from build123d import *

# Parameters (mm, degrees)
F0_W     = 150
F0_H     = 194.7
F0_R     = 2
F1_DEPTH = 2.032
F2_W     = 20
F2_H     = 2
F3_DEPTH = 35.71875
F4_DEPTH = 66.675
F5_R     = 2
F6_DEPTH = 2
F7_W     = 2.032
F7_H     = 20
F8_DEPTH = 39
F9_R     = 2
F10_R    = 1.99999
F11_R    = 0.5


# Not quite as in the source:
# - a fillet or chamfer is up to 0.001 mm smaller than in the source, because OpenCascade refuses the exact size


with BuildPart() as f1:
    # F0 (on Front) → F1 (new body)
    with BuildSketch(Plane.XZ):
        with Locations((0, -42.35)):
            Rectangle(F0_W, F0_H)
        with Locations((-50, -50)):
            Circle(F0_R, mode=Mode.SUBTRACT)
        with Locations((50, -50)):
            Circle(F0_R, mode=Mode.SUBTRACT)
        with Locations((-37.5, -37.5)):
            Circle(F0_R, mode=Mode.SUBTRACT)
        with Locations((-50, 50)):
            Circle(F0_R, mode=Mode.SUBTRACT)
        with Locations((-37.5, 37.5)):
            Circle(F0_R, mode=Mode.SUBTRACT)
        with Locations((37.5, -37.5)):
            Circle(F0_R, mode=Mode.SUBTRACT)
        with Locations((37.5, 37.5)):
            Circle(F0_R, mode=Mode.SUBTRACT)
        with Locations((50, 50)):
            Circle(F0_R, mode=Mode.SUBTRACT)
    extrude(amount=F1_DEPTH)

    # F2 (on Right) → F3 (join, symmetric)
    with BuildSketch(Plane.YZ):
        with Locations((-12.032, -138.7)):
            Rectangle(F2_W, F2_H)
    extrude(amount=F3_DEPTH, both=True)

    # F2 (on Right) → F4 (join, symmetric)
    with BuildSketch(Plane.YZ):
        Polygon((-24.032, -139.7), (-22.032, -139.7), (-22.032, -137.7), (-22.032, -109.7), (-24.032, -109.7), align=None)
    extrude(amount=F4_DEPTH, both=True)

    # F5 (on face) → F6 (cut, through all)
    with BuildSketch(Plane.XZ.offset(24.032)):
        with Locations((-50.8, -114.7)):
            Circle(F5_R)
        with Locations((-23.6466728747, -130.575)):
            Circle(F5_R)
        with Locations((50.8, -114.7)):
            Circle(F5_R)
        with Locations((23.6466728747, -130.575)):
            Circle(F5_R)
    extrude(amount=-F6_DEPTH, mode=Mode.SUBTRACT)

    # F7 (on face) → F8 (join)
    with BuildSketch(Plane.XY.offset(-137.7)):
        with Locations((-34.70275, -12.032)):
            Rectangle(F7_W, F7_H)
        with Locations((34.70275, -12.032)):
            Rectangle(F7_W, F7_H)
    extrude(amount=F8_DEPTH)

    # F9
    f9_edges = [f1.edges().sort_by_distance(p)[0] for p in [
        (35.71875, -2.032, -119.2),
        (35.71875, -22.032, -124.7),
        (-35.71875, -2.032, -119.2),
        (-35.71875, -22.032, -124.7),
    ]]
    fillet(f9_edges, radius=F9_R)

    # F10 (radius 2 in the source; OpenCascade refuses exactly that, so slightly less here)
    f10_edges = [f1.edges().sort_by_distance(p)[0] for p in [
        (0, 0, -139.7),
        (0, -24.032, -139.7),
    ]]
    fillet(f10_edges, radius=F10_R)

    # F11
    f11_edges = [f1.edges().sort_by_distance(p)[0] for p in [
        (-35.71875, -12.032, -139.7),
        (35.71875, -12.032, -139.7),
        (33.68675, -12.032, -137.7),
        (-33.68675, -12.032, -137.7),
    ]]
    fillet(f11_edges, radius=F11_R)


solid = f1.part
Design review of the part built by this model. Coordinates are the model's own, in mm. A direction names the side the tool comes from. Round coordinates to 2 decimals unless told otherwise and drop trailing zeros. Write each loop counter-clockwise with the first axis right and the second up, starting at its lowest first coordinate (ties: lowest second). Pieces come first, ordered by that corner, then holes. Notation, with made-up numbers: (-28, 77.25) -> (18, 77.25) arc R22 ccw to (18, 108.25) -> close; hole circle Ø9 at (-28, 76). An arc over 180 degrees is marked (long way). One line per item, written item: value. Start each with the question number.
Q1. The part is to be moulded in two halves that separate along Y. For faces 6 (the face through (0, -12, -137.7)), 7 (the face through (1, -24.032, -124)), 8 (the face through (35, -12, -98.7)), say which applies: pulls with the +Y half, pulls with the -Y half, needs draft (parallel to the pull), parting line crosses it, or undercut.
Q2. Add section B-B (z = 37.5). Give the boundary of the cut face in (x, y).
Q3. Add section C-C (x = -15.5). Give the boundary of the cut face in (y, z), then the cut area to 3 significant figures.
Q4. Insertion check: P1, Ø4.5, axis at x = 37.5, z = -37.5, coming from the -Y side; P2, Ø1, axis at y = -23.5, z = -121.5, coming from the -X side (3 decimals); P3, Ø1.6, axis at x = -35, z = -103, coming from the -Y side; P4, Ø3, axis at x = -50, z = -50, coming from the +Y side. Each pin has a flat end and moves straight along its axis. Give the tip position at first contact, or say it passes through.
Q5. To check wall thickness, follow probe 1 along Z at (x, y) = (37.5, -1.5); probe 2 along Z at (x, y) = (50, -1.15); probe 3 along X at (y, z) = (-8.75, -103). State the ranges of each line that lie inside material, in increasing order.
Q6. Tool access review of faces 1 (the face through (52, -22.032, -125)), 2 (the face through (24.57, -23.05, -132.35)), 3 (the face through (-52, -22.032, -125)), 4 (the face through (-35, -12, -98.7)), 5 (the face through (-33.687, -12, -118)): name each direction out of +Z, -Z, +X, -X, +Y, -Y from which nothing blocks a thin tool from reaching the whole face with its end or side.
Q7. Add section D-D (y = -10.25). Give the boundary of the cut face in (x, z).
Q8. Add section A-A (z = -114.7). Give the boundary of the cut face in (x, y) (3 decimals).
Response:
1. face 6: undercut
1. face 7: pulls with the -Y half
1. face 8: needs draft
2. outline: (-75, -2.03) -> (-39.5, -2.03) -> (-39.5, 0) -> (-75, 0) -> close; (-35.5, -2.03) -> (35.5, -2.03) -> (35.5, 0) -> (-35.5, 0) -> close; (39.5, -2.03) -> (75, -2.03) -> (75, 0) -> (39.5, 0) -> close
3. outline: (-24.03, -137.7) arc R2 ccw to (-22.03, -139.7) -> (-2, -139.7) arc R2 ccw to (0, -137.7) -> (0, 55) -> (-2.03, 55) -> (-2.03, -137.7) -> (-22.03, -137.7) -> (-22.03, -109.7) -> (-24.03, -109.7) -> close
3. area: 494 mm^2
4. P1: stops at y = -2.03
4. P2: stops at x = -66.675
4. P3: stops at y = -22.03
4. P4: passes through
5. probe 1: z = -139.63 to -39.5, -35.5 to 35.5, 39.5 to 55
5. probe 2: z = -139.51 to -52, -48 to 48, 52 to 55
5. probe 3: x = -35.72 to -33.69, 33.69 to 35.72
6. face 1: +Z, -Z, +X
6. face 2: -Y
6. face 3: +Z, -Z, -X
6. face 4: +Z, +X, -X, -Y
6. face 5: +Z
7. outline: (-35.72, -139.2) arc R0.5 ccw to (-35.22, -139.7) -> (35.22, -139.7) arc R0.5 ccw to (35.72, -139.2) -> (35.72, -98.7) -> (33.69, -98.7) -> (33.69, -137.2) arc R0.5 cw to (33.19, -137.7) -> (-33.19, -137.7) arc R0.5 cw to (-33.69, -137.2) -> (-33.69, -98.7) -> (-35.72, -98.7) -> close
8. outline: (-75, -2.032) -> (-37.719, -2.032) arc R2 cw to (-35.719, -4.032) -> (-35.719, -20.032) arc R2 cw to (-37.719, -22.032) -> (-48.8, -22.032) -> (-48.8, -24.032) -> (48.8, -24.032) -> (48.8, -22.032) -> (37.719, -22.032) arc R2 cw to (35.719, -20.032) -> (35.719, -4.032) arc R2 cw to (37.719, -2.032) -> (75, -2.032) -> (75, 0) -> (-75, 0) -> close; (-66.675, -24.032) -> (-52.8, -24.032) -> (-52.8, -22.032) -> (-66.675, -22.032) -> close; (52.8, -24.032) -> (66.675, -24.032) -> (66.675, -22.032) -> (52.8, -22.032) -> close; hole (-33.687, -22.032) -> (33.687, -22.032) -> (33.687, -2.032) -> (-33.687, -2.032) -> close
